from build123d import *

# Parameters (mm, degrees)
F0_W     = 32
F0_H     = 46
F0_R     = 1.6
F0_R_2   = 4
F1_DEPTH = 25
F3_DEPTH = 35
F0_R_3   = 3
F4_DEPTH = 23
F5_DEPTH = 40


with BuildPart() as f1:
    # F0 (on Top) → F1 (new body)
    with BuildSketch(Plane.XY):
        with Locations((16, 23)):
            Rectangle(F0_W, F0_H)
        with Locations((6.6, 6.6)):
            Circle(F0_R, mode=Mode.SUBTRACT)
        with Locations((25.4, 6.6)):
            Circle(F0_R, mode=Mode.SUBTRACT)
        with Locations((6.6, 39.4)):
            Circle(F0_R, mode=Mode.SUBTRACT)
        with Locations((16, 31)):
            Circle(F0_R_2, mode=Mode.SUBTRACT)
        with Locations((25.4, 39.4)):
            Circle(F0_R, mode=Mode.SUBTRACT)
    extrude(amount=F1_DEPTH)

    # F2 (on face) → F3 (join)
    with BuildSketch(Plane.XZ):
        with BuildLine():
            ThreePointArc((24.63325, 0), (28.573528, 4.325451), (30, 10))
            ThreePointArc((30, 10), (12.325451, 20.573528), (11.36675, 0))
            Line((11.36675, 0), (24.63325, 0))
        make_face()
        with BuildLine():
            Line((24.63325, 0), (11.36675, 0))
            ThreePointArc((11.36675, 0), (18, -2), (24.63325, 0))
        make_face()
    extrude(amount=F3_DEPTH)

    # F0 (on Top) → F4 (join)
    with BuildSketch(Plane.XY):
        with Locations((16, 31)):
            Circle(F0_R_2)
        with Locations((16, 31)):
            Circle(F0_R_3, mode=Mode.SUBTRACT)
    extrude(amount=F4_DEPTH)

    # F0 (on Top) → F5 (join)
    with BuildSketch(Plane.XY):
        with Locations((16, 31)):
            Circle(F0_R_3)
    extrude(amount=F5_DEPTH)


solid = f1.part
For this review, take the finished solid that the model builds, in its own axes (mm). A direction names the side the tool comes from. Round coordinates to 2 decimals unless told otherwise and drop trailing zeros. Loops run counter-clockwise (first coordinate to the right, second up) from the corner with the lowest first, then second, coordinate; pieces in that order, holes last. Notation, with made-up numbers: (39.25, 23) - (92.25, 23) arc R29 cw to (92.25, 60) - close; hole circle Ø5 at (9, 69). An arc over 180 degrees is marked (long way). One line per item, written item: value. Start each with the question number.
Item 1: The part is to be moulded in two halves that separate along X. For faces 1 (the flat face through (0, 23, 12)), 2 (the flat face through (18, 0, -1)), 3 (the flat face through (17, 34, 23)), say which applies: +X half, -X half, draft (parallel to the pull), parting line (faces both ways), or undercut.
Item 2: Clearance check with flat-ended pins moving along their axes: pin 1 Ø16 at (x, y) = (13.5, 14) entering from -Z; pin 2 Ø4 at (x, y) = (6.6, 39.4) entering from +Z; pin 3 Ø1.6 at (x, z) = (17.5, -1) entering from +Y; pin 4 Ø12 at (y, z) = (5, 23.5) entering from -X. State where each tip first meets the part, or that it passes through.
Item 3: For faces 4 (the cylindrical face through (15.479, 34.966, 23.986)), 5 (the flat face through (16, 23, 0)), 6 (the flat face through (8.7, 0, 17.9)), list the 3-axis set-ups (+Z, -Z, +X, -X, +Y, -Y) from which the entire face can be reached by the end or side of a thin tool; tool diameter is ignored.
Item 4: Take a section at B-B (y = 39.4). Give the boundary of the cut face in (x, z).
Item 5: For L1, parallel to Y at x = 16, z = 24.5; L2, parallel to Y at x = 6.6, z = 15.75; L3, parallel to Z at x = 27, y = 17.5, list the stretches that pass through material, from the lowest coordinate up.
Item 6: Take a section at D-D (x = 18). Give the boundary of the cut face in (y, z).
Item 7: Take a section at A-A (z = 24). Give the boundary of the cut face in (x, y), plus the area to 3 significant figures.
Item 8: Take a section at C-C (z = 19.5). Give the boundary of the cut face in (x, y).
Answer below:
1. face 1: -X half
1. face 2: draft
1. face 3: undercut
2. pin 1: stops at z = 0
2. pin 2: stops at z = 25
2. pin 3: stops at y = 0
2. pin 4: stops at x = 0
3. face 4: +Z
3. face 5: -Z, +X, -X, +Y
3. face 6: -Y
4. outline: (0, 0) - (5, 0) - (5, 25) - (0, 25) - close; (8.2, 0) - (23.8, 0) - (23.8, 25) - (8.2, 25) - close; (27, 0) - (32, 0) - (32, 25) - (27, 25) - close
5. L1: y = 0 to 27, 28 to 34, 35 to 46
5. L2: y = 0 to 5, 8.2 to 37.8, 41 to 46
5. L3: z = 0 to 25
6. outline: (-35, -2) - (0, -2) - (0, 0) - (46, 0) - (46, 25) - (34.46, 25) - (34.46, 23) - (33.24, 23) - (33.24, 40) - (28.76, 40) - (28.76, 23) - (27.54, 23) - (27.54, 25) - (0, 25) - (0, 22) - (-35, 22) - close
7. outline: (0, 0) - (32, 0) - (32, 46) - (0, 46) - close; circle Ø6 at (16, 31); hole circle Ø3.2 at (6.6, 6.6); hole circle Ø3.2 at (6.6, 39.4); hole circle Ø8 at (16, 31); hole circle Ø3.2 at (25.4, 6.6); hole circle Ø3.2 at (25.4, 39.4)
7. area: 1,420 mm2
8. outline: (0, 0) - (10.67, 0) - (10.67, -35) - (25.33, -35) - (25.33, 0) - (32, 0) - (32, 46) - (0, 46) - close; hole circle Ø3.2 at (6.6, 6.6); hole circle Ø3.2 at (6.6, 39.4); hole circle Ø3.2 at (25.4, 6.6); hole circle Ø3.2 at (25.4, 39.4)
